from build123d import *

# Parameters (mm, degrees)
BOSS_EXTRUDE1_DEPTH = 36
CUT_EXTRUDE1_START  = -5.5
SKETCH2_R           = 17
CUT_EXTRUDE1_DEPTH  = 11.5
FILLET1_R           = 10
SKETCH3_R           = 11
CUT_EXTRUDE2_DEPTH  = 5.6
SKETCH4_R           = 1.25
CUT_EXTRUDE3_DEPTH  = 13.4
SKETCH5_R           = 2
CUT_EXTRUDE4_DEPTH  = 156.152860109
CUT_EXTRUDE5_START  = -2.5
SKETCH6_R           = 3.5
SKETCH6_R_2         = 2
CUT_EXTRUDE5_DEPTH  = 2.5
CUT_EXTRUDE6_START  = -12.5
CUT_EXTRUDE6_DEPTH  = 7.5
LPATTERN1_COUNT     = 2
LPATTERN1_PITCH     = 20.5
SKETCH8_R           = 2
CUT_EXTRUDE7_DEPTH  = 157.346570157
FILLET2_R           = 9
CUT_EXTRUDE8_DEPTH  = 13.5
BOSS_EXTRUDE2_START = 2.039261455
BOSS_EXTRUDE2_DEPTH = 2.039261455
SKETCH15_R          = 2
CUT_EXTRUDE9_DEPTH  = 157.828681726
SKETCH17_R          = 3.5
SKETCH17_R_2        = 2
CUT_EXTRUDE10_DEPTH = 3
FILLET4_R           = 6
CUT_EXTRUDE11_DEPTH = 158.606994039


with BuildPart() as part:
    # Sketch1 → Boss-Extrude1 (new body)
    with BuildSketch(Plane(origin=(0, 0, 0), x_dir=(1, 0, 0), z_dir=(0, 1, 0))):
        with BuildLine():
            ThreePointArc((7.5, 144), (0, 151.5), (-7.5, 144))
            Line((-7.5, 144), (-14, 0))
            ThreePointArc((-14, 0), (0, -14), (14, 0))
            Line((14, 0), (7.5, 144))
        make_face()
    extrude(amount=BOSS_EXTRUDE1_DEPTH)

    # Sketch2 → Cut-Extrude1 (cut)
    with BuildSketch(Plane(origin=(0, 36, 0), x_dir=(1, 0, 0), z_dir=(0, 1, 0)).offset(CUT_EXTRUDE1_START)):
        Circle(SKETCH2_R)
    extrude(amount=-CUT_EXTRUDE1_DEPTH, mode=Mode.SUBTRACT)

    # Fillet1
    fillet1_edges = [part.edges().sort_by_distance(p)[0] for p in [
        (-13.535741066, 24.75, -10.28512099),
        (13.535741066, 24.75, -10.28512099),
    ]]
    fillet(fillet1_edges, radius=FILLET1_R)

    # Sketch3 → Cut-Extrude2 (cut)
    with BuildSketch(Plane.XZ):
        with Locations(Location((0, 0, 0), (0, 0, 270))):
            Circle(SKETCH3_R)
    extrude(amount=-CUT_EXTRUDE2_DEPTH, mode=Mode.SUBTRACT)

    # Sketch4 → Cut-Extrude3 (cut)
    with BuildSketch(Plane.XZ.offset(-5.6)):
        with Locations(Location((0, -7.25, 0), (0, 0, 270))):
            Circle(SKETCH4_R)
        with Locations(Location((-7.25, 0, 0), (0, 0, 270))):
            Circle(SKETCH4_R)
        with Locations(Location((0, 7.25, 0), (0, 0, 270))):
            Circle(SKETCH4_R)
        with Locations(Location((7.25, 0, 0), (0, 0, 270))):
            Circle(SKETCH4_R)
    extrude(amount=-CUT_EXTRUDE3_DEPTH, mode=Mode.SUBTRACT)

    # Sketch5 → Cut-Extrude4 (cut, through all)
    with BuildSketch(Plane.XZ.offset(-5.6)):
        with Locations(Location((0, 0, 0), (0, 0, 270))):
            Circle(SKETCH5_R)
    extrude(amount=-CUT_EXTRUDE4_DEPTH, mode=Mode.SUBTRACT)

    # Sketch6 → Cut-Extrude5 (cut)
    with BuildSketch(Plane(origin=(0, 36, 0), x_dir=(1, 0, 0), z_dir=(0, 1, 0)).offset(CUT_EXTRUDE5_START)):
        with Locations(Location((0, 0, 0), (0, 0, 270))):
            Circle(SKETCH6_R)
        with Locations(Location((0, 0, 0), (0, 0, 270))):
            Circle(SKETCH6_R_2, mode=Mode.SUBTRACT)
    extrude(amount=CUT_EXTRUDE5_DEPTH, mode=Mode.SUBTRACT)

    # Sketch7 → Cut-Extrude6 (cut)
    with BuildSketch(Plane(origin=(0, 36, 0), x_dir=(1, 0, 0), z_dir=(0, 1, 0)).offset(CUT_EXTRUDE6_START)):
        with BuildLine():
            Line((-7.5, 144), (-8.177083333, 129))
            Line((-8.177083333, 129), (8.177083333, 129))
            Line((8.177083333, 129), (7.5, 144))
            ThreePointArc((7.5, 144), (0, 151.5), (-7.5, 144))
        make_face()
    cut_extrude6 = extrude(amount=CUT_EXTRUDE6_DEPTH, mode=Mode.SUBTRACT)

    # LPattern1: Cut-Extrude6 ×2
    with Locations(*[(0, -i * LPATTERN1_PITCH, 0) for i in range(1, LPATTERN1_COUNT)]):
        add(cut_extrude6, mode=Mode.SUBTRACT)

    # Sketch8 → Cut-Extrude7 (cut, through all)
    with BuildSketch(Plane.XZ):
        with Locations(Location((0, -144, 0), (0, 0, 90))):
            Circle(SKETCH8_R)
    extrude(amount=-CUT_EXTRUDE7_DEPTH, mode=Mode.SUBTRACT)

    # Fillet2
    # the kernel refuses this fillet: 9 mm, written as the material it takes off along each edge
    with BuildSketch(Plane(origin=(-8.177083333, 1.992714572, -129), x_dir=(1, 0, 0), z_dir=(0, 1, 0))) as fillet2_piece_1_section:
        with BuildLine():
            CenterArc((FILLET2_R * 0.955879352349, -FILLET2_R), FILLET2_R, 90, 87.415486554)
            Line((-FILLET2_R * 0.0431034421745, -FILLET2_R * 0.954907026636), (0, 0))
            Line((0, 0), (FILLET2_R * 0.955879352349, 0))
        make_face()
    fillet2_piece_1 = extrude(amount=50.514570856, mode=Mode.PRIVATE)
    fillet2_piece_1 = split(fillet2_piece_1, bisect_by=Plane(origin=(-8.177083333, 3, -129), z_dir=(0, 1, 0)), keep=Keep.TOP, mode=Mode.PRIVATE)
    fillet2_piece_1 = split(fillet2_piece_1, bisect_by=Plane(origin=(-8.177083333, 10.5, -129), z_dir=(0, -1, 0)), keep=Keep.TOP, mode=Mode.PRIVATE)
    add(fillet2_piece_1, mode=Mode.SUBTRACT)
    with BuildSketch(Plane(origin=(-8.177083333, 23.5, -129), x_dir=(1, 0, 0), z_dir=(0, 1, 0)), Plane(origin=(-8.177083333, 3, -129), x_dir=(1, 0, 0), z_dir=(0, 1, 0)), Plane(origin=(8.177083333, 23.5, -129), x_dir=(0.04509297336389057, 0, 0.9989827945231107), z_dir=(0, 1, 0)), Plane(origin=(8.177083333, 3, -129), x_dir=(0.04509297336389057, 0, 0.9989827945231107), z_dir=(0, 1, 0))) as fillet2_piece_2:
        with BuildLine():
            CenterArc((FILLET2_R * 0.955879352349, -FILLET2_R), FILLET2_R, 90, 87.415486554)
            Line((-FILLET2_R * 0.0431034421745, -FILLET2_R * 0.954907026636), (0, 0))
            Line((0, 0), (FILLET2_R * 0.955879352349, 0))
        make_face()
    extrude(amount=7.5, mode=Mode.SUBTRACT)
    with BuildSketch(Plane(origin=(-8.177083333, -18.507285428, -129), x_dir=(1, 0, 0), z_dir=(0, 1, 0))) as fillet2_piece_3_section:
        with BuildLine():
            CenterArc((FILLET2_R * 0.955879352349, -FILLET2_R), FILLET2_R, 90, 87.415486554)
            Line((-FILLET2_R * 0.0431034421745, -FILLET2_R * 0.954907026636), (0, 0))
            Line((0, 0), (FILLET2_R * 0.955879352349, 0))
        make_face()
    fillet2_piece_3 = extrude(amount=50.514570856, mode=Mode.PRIVATE)
    fillet2_piece_3 = split(fillet2_piece_3, bisect_by=Plane(origin=(-8.177083333, 23.5, -129), z_dir=(0, 1, 0)), keep=Keep.TOP, mode=Mode.PRIVATE)
    fillet2_piece_3 = split(fillet2_piece_3, bisect_by=Plane(origin=(-8.177083333, 31, -129), z_dir=(0, -1, 0)), keep=Keep.TOP, mode=Mode.PRIVATE)
    add(fillet2_piece_3, mode=Mode.SUBTRACT)
    with BuildSketch(Plane(origin=(8.177083333, 1.992714572, -129), x_dir=(0.04509297336389057, 0, 0.9989827945231107), z_dir=(0, 1, 0))) as fillet2_piece_4_section:
        with BuildLine():
            CenterArc((FILLET2_R * 0.955879352349, -FILLET2_R), FILLET2_R, 90, 87.415486554)
            Line((-FILLET2_R * 0.0431034421745, -FILLET2_R * 0.954907026636), (0, 0))
            Line((0, 0), (FILLET2_R * 0.955879352349, 0))
        make_face()
    fillet2_piece_4 = extrude(amount=50.514570856, mode=Mode.PRIVATE)
    fillet2_piece_4 = split(fillet2_piece_4, bisect_by=Plane(origin=(8.177083333, 3, -129), z_dir=(0, 1, 0)), keep=Keep.TOP, mode=Mode.PRIVATE)
    fillet2_piece_4 = split(fillet2_piece_4, bisect_by=Plane(origin=(8.177083333, 10.5, -129), z_dir=(0, -1, 0)), keep=Keep.TOP, mode=Mode.PRIVATE)
    add(fillet2_piece_4, mode=Mode.SUBTRACT)
    with BuildSketch(Plane(origin=(8.177083333, -18.507285428, -129), x_dir=(0.04509297336389057, 0, 0.9989827945231107), z_dir=(0, 1, 0))) as fillet2_piece_5_section:
        with BuildLine():
            CenterArc((FILLET2_R * 0.955879352349, -FILLET2_R), FILLET2_R, 90, 87.415486554)
            Line((-FILLET2_R * 0.0431034421745, -FILLET2_R * 0.954907026636), (0, 0))
            Line((0, 0), (FILLET2_R * 0.955879352349, 0))
        make_face()
    fillet2_piece_5 = extrude(amount=50.514570856, mode=Mode.PRIVATE)
    fillet2_piece_5 = split(fillet2_piece_5, bisect_by=Plane(origin=(8.177083333, 23.5, -129), z_dir=(0, 1, 0)), keep=Keep.TOP, mode=Mode.PRIVATE)
    fillet2_piece_5 = split(fillet2_piece_5, bisect_by=Plane(origin=(8.177083333, 31, -129), z_dir=(0, -1, 0)), keep=Keep.TOP, mode=Mode.PRIVATE)
    add(fillet2_piece_5, mode=Mode.SUBTRACT)

    # Sketch9 → Cut-Extrude8 (cut)
    with BuildSketch(Plane.XZ):
        with BuildLine():
            Line((8.977561109, -111.266338499), (-8.977561109, -111.266338499))
            Line((-8.977561109, -111.266338499), (-13.265142213, -16.279926353))
            ThreePointArc((-13.265142213, -16.279926353), (0, -21), (13.265142213, -16.279926353))
            Line((13.265142213, -16.279926353), (8.977561109, -111.266338499))
        make_face()
    extrude(amount=-CUT_EXTRUDE8_DEPTH, mode=Mode.SUBTRACT)

    # Sketch10 → Boss-Extrude2 (add)
    with BuildSketch(Plane.XZ.offset(BOSS_EXTRUDE2_START)):
        with BuildLine():
            Line((7.5, -144), (8.977561109, -111.266338499))
            Line((8.977561109, -111.266338499), (-8.977561109, -111.266338499))
            Line((-8.977561109, -111.266338499), (-7.5, -144))
            ThreePointArc((-7.5, -144), (0, -151.5), (7.5, -144))
        make_face()
    extrude(amount=-BOSS_EXTRUDE2_DEPTH)

    # Sketch15 → Cut-Extrude9 (cut, through all)
    with BuildSketch(Plane(origin=(0, 36, 0), x_dir=(1, 0, 0), z_dir=(0, 1, 0))):
        with Locations(Location((0, 144, 0), (0, 0, 270))):
            Circle(SKETCH15_R)
    extrude(amount=-CUT_EXTRUDE9_DEPTH, mode=Mode.SUBTRACT)

    # Sketch17 → Cut-Extrude10 (cut)
    with BuildSketch(Plane.XZ.offset(2.039261455)):
        with Locations(Location((0, -144, 0), (0, 0, 270))):
            Circle(SKETCH17_R)
        with Locations(Location((0, -144, 0), (0, 0, 270))):
            Circle(SKETCH17_R_2, mode=Mode.SUBTRACT)
    extrude(amount=-CUT_EXTRUDE10_DEPTH, mode=Mode.SUBTRACT)

    # Fillet3: read off the stored shape, not the designer's step
    # Fillet3 outline → Fillet3 (revolve, cut)
    with BuildSketch(Plane.XY):
        with BuildLine():
            ThreePointArc((21, 10), (18.071067812, 2.928932188), (11, 0))
            Line((11, 0), (21, 0))
            Line((21, 0), (21, 10))
        make_face()
    revolve(axis=Axis((0, 0, 0), (0, 1, 0)), mode=Mode.SUBTRACT)

    # Fillet4
    fillet4_edges = [part.edges().sort_by_distance(p)[0] for p in [
        (0, 13.5, -21),
        (0, 13.5, -111.266338499),
        (0, -2.039261455, -111.266338499),
    ]]
    fillet(fillet4_edges, radius=FILLET4_R)

    # Sketch18 → Cut-Extrude11 (cut, through all)
    with BuildSketch(Plane(origin=(-13.971532733, 0, -0.630659464), x_dir=(-0.04509297336389045, 0, 0.9989827945231107), z_dir=(-0.9989827945231108, 0, -0.04509297336389045))):
        with BuildLine():
            Line((-79.983553336, 21.75), (-79.983553336, 27.75))
            ThreePointArc((-79.983553336, 27.75), (-79.10487368, 29.871320344), (-76.983553336, 30.75))
            Line((-76.983553336, 30.75), (-66.983553336, 30.75))
            ThreePointArc((-66.983553336, 30.75), (-64.862232993, 29.871320344), (-63.983553336, 27.75))
            Line((-63.983553336, 27.75), (-63.983553336, 21.75))
            ThreePointArc((-63.983553336, 21.75), (-64.862232993, 19.628679656), (-66.983553336, 18.75))
            Line((-66.983553336, 18.75), (-76.983553336, 18.75))
            ThreePointArc((-76.983553336, 18.75), (-79.10487368, 19.628679656), (-79.983553336, 21.75))
        make_face()
        with BuildLine():
            Line((-106.983553336, 18.75), (-96.983553336, 18.75))
            ThreePointArc((-96.983553336, 18.75), (-94.862232993, 19.628679656), (-93.983553336, 21.75))
            Line((-93.983553336, 21.75), (-93.983553336, 27.75))
            ThreePointArc((-93.983553336, 27.75), (-94.862232993, 29.871320344), (-96.983553336, 30.75))
            Line((-96.983553336, 30.75), (-106.983553336, 30.75))
            ThreePointArc((-106.983553336, 30.75), (-109.10487368, 29.871320344), (-109.983553336, 27.75))
            Line((-109.983553336, 27.75), (-109.983553336, 21.75))
            ThreePointArc((-109.983553336, 21.75), (-109.10487368, 19.628679656), (-106.983553336, 18.75))
        make_face()
        with BuildLine():
            Line((-49.983553336, 21.75), (-49.983553336, 27.75))
            ThreePointArc((-49.983553336, 27.75), (-49.10487368, 29.871320344), (-46.983553336, 30.75))
            Line((-46.983553336, 30.75), (-36.983553336, 30.75))
            ThreePointArc((-36.983553336, 30.75), (-34.862232993, 29.871320344), (-33.983553336, 27.75))
            Line((-33.983553336, 27.75), (-33.983553336, 21.75))
            ThreePointArc((-33.983553336, 21.75), (-34.862232993, 19.628679656), (-36.983553336, 18.75))
            Line((-36.983553336, 18.75), (-46.983553336, 18.75))
            ThreePointArc((-46.983553336, 18.75), (-49.10487368, 19.628679656), (-49.983553336, 21.75))
        make_face()
    extrude(amount=-CUT_EXTRUDE11_DEPTH, mode=Mode.SUBTRACT)


solid = part.part
Geometry: final body of the model. Coordinates: model frame, mm. A direction names the side the tool comes from. Round coordinates to 2 decimals unless told otherwise and drop trailing zeros. Loops run counter-clockwise (first coordinate to the right, second up) from the corner with the lowest first, then second, coordinate; pieces in that order, holes last. Notation, with made-up numbers: M -30.5,21.25 L -17.5,21.25 A17 ccw -17.5,42.25 Z; hole C 25.25,82 d7. An arc over 180 degrees is marked long. Put each result on its own line as item: value. Start each with the question number.
(1) Set-up query: faces 1 (the face through (-0.092, 29.895, -64.956)), 2 (the face through (-0.015, 29.895, -109.193)), 3 (the face through (1.05, -0.56, -147.34)), 4 (the face through (-2, 33.5, 2)). Return all of +Z, -Z, +X, -X, +Y, -Y with unobstructed straight access to the full face (end or side cutting, diameter ignored); none if empty.
(2) Section query A-A (z = -45). Return loops of the section in (x, y).
(3) Material intervals for line 1 along X through (y, z) = (34, 0); line 2 along X through (y, z) = (32.75, 0); line 3 along Z through (x, y) = (-3.75, 27), sorted ascending. Write a range as [from, to].
(4) Contact query for flat-ended pins moving along their axis: pin 1 Ø5 at (x, z) = (7.5, -32) entering from -Y; pin 2 Ø9 at (x, z) = (0, 0) entering from -Y; pin 3 Ø4.5 at (x, z) = (0, -144) entering from -Y; pin 4 Ø3 at (x, z) = (0, 0) entering from -Y. Output: stop coordinate, or through.
(5) Draft query along X for faces 5 (the face through (-2, 12, 0)), 6 (the face through (0, 30.75, -72)), 7 (the face through (0.16, 33.47, -151.5)). Return one class per face: +X half, -X half, draft (parallel to the pull), parting line (faces both ways), or undercut.
Findings below:
1. face 1: +X
1. face 2: -X
1. face 3: -Y
1. face 4: +Y
2. outline: M -11.97,13.5 L 11.97,13.5 L 11.97,18.75 L -11.97,18.75 Z; M -11.97,30.75 L 11.97,30.75 L 11.97,36 L -11.97,36 Z
3. line 1: x = [-14, -3.5], [3.5, 14]
3. line 2: x = [-14, -2], [2, 14]
3. line 3: z = [-127.97, -110.26], [-94.25, -80.23], [-64.22, -50.2], [-34.19, -16.9]
4. pin 1: stops at y = 13.5
4. pin 2: stops at y = 5.6
4. pin 3: stops at y = 0.96
4. pin 4: passes through
5. face 5: undercut
5. face 6: draft
5. face 7: parting line
